```python
from build123d import *

# Parameters (mm, degrees)
CROQUIS1_W              = 70
CROQUIS1_H              = 117
SALIENTE_EXTRUIR1_DEPTH = 5
CROQUIS2_W              = 70
CROQUIS2_H              = 11.75
SALIENTE_EXTRUIR2_DEPTH = 40
CROQUIS5_R              = 1
CORTAR_EXTRUIR3_DEPTH   = 118
CROQUIS3_W              = 43.35
CROQUIS3_H              = 81.55
CORTAR_EXTRUIR1_DEPTH   = 10
SALIENTE_EXTRUIR4_DEPTH = 40
CROQUIS7_R              = 1.25
CROQUIS7_W              = 60
CROQUIS7_H              = 11.191024472
CORTAR_EXTRUIR5_DEPTH   = 71
CROQUIS9_W              = 50
CROQUIS9_H              = 20
CORTAR_EXTRUIR6_DEPTH   = 118
CROQUIS11_W             = 5
CROQUIS11_H             = 45
CROQUIS11_H_2           = 15
CROQUIS11_H_3           = 10
SALIENTE_EXTRUIR5_DEPTH = 20
CROQUIS12_W             = 42.5
CROQUIS12_H             = 15
CORTAR_EXTRUIR7_DEPTH   = 20
CROQUIS13_W             = 5
CROQUIS13_H             = 31.75
SALIENTE_EXTRUIR6_DEPTH = 5
CROQUIS14_W             = 55
CROQUIS14_H             = 31.75
SALIENTE_EXTRUIR7_DEPTH = 5


with BuildPart() as part:
    # Croquis1 → Saliente-Extruir1 (new body)
    with BuildSketch(Plane(origin=(0, 0, 0), x_dir=(1, 0, 0), z_dir=(0, 1, 0))):
        Rectangle(CROQUIS1_W, CROQUIS1_H)
    extrude(amount=SALIENTE_EXTRUIR1_DEPTH)

    # Croquis2 → Saliente-Extruir2 (add)
    with BuildSketch(Plane(origin=(0, 5, 0), x_dir=(1, 0, 0), z_dir=(0, 1, 0))):
        with Locations((0, 52.625)):
            Rectangle(CROQUIS2_W, CROQUIS2_H)
        with Locations((0, -52.625)):
            Rectangle(CROQUIS2_W, CROQUIS2_H)
    extrude(amount=SALIENTE_EXTRUIR2_DEPTH)

    # Croquis5 → Cortar-Extruir3 (cut, through all)
    with BuildSketch(Plane(origin=(0, 0, -58.5), x_dir=(-1, 0, 0), z_dir=(0, 0, -1))):
        with Locations((5, 35)):
            Circle(CROQUIS5_R)
    extrude(amount=-CORTAR_EXTRUIR3_DEPTH, mode=Mode.SUBTRACT)

    # Croquis3 → Cortar-Extruir1 (cut)
    with BuildSketch(Plane(origin=(0, 5, 0), x_dir=(1, 0, 0), z_dir=(0, 1, 0))):
        with Locations((0, 10.775)):
            Rectangle(CROQUIS3_W, CROQUIS3_H)
    extrude(amount=-CORTAR_EXTRUIR1_DEPTH, mode=Mode.SUBTRACT)

    # Croquis8 → Saliente-Extruir4 (add)
    with BuildSketch(Plane(origin=(0, 5, 0), x_dir=(1, 0, 0), z_dir=(0, 1, 0))):
        Polygon((35, -46.75), (35, 46.75), (21.675, 46.75), (21.675, -30), (-21.675, -30), (-21.675, 46.75), (-35, 46.75), (-35, -46.75), align=None)
    extrude(amount=SALIENTE_EXTRUIR4_DEPTH)

    # Croquis7 → Cortar-Extruir5 (cut, through all)
    with BuildSketch(Plane.ZY.offset(35)):
        with Locations((-9.99, 32.49)):
            Circle(CROQUIS7_R)
        with Locations((9.99, 32.49)):
            Circle(CROQUIS7_R)
        with Locations((9.99, 12.51)):
            Circle(CROQUIS7_R)
        with Locations((-9.99, 12.51)):
            Circle(CROQUIS7_R)
        with Locations((-10.75, 23.745325958)):
            Rectangle(CROQUIS7_W, CROQUIS7_H)
    extrude(amount=-CORTAR_EXTRUIR5_DEPTH, mode=Mode.SUBTRACT)

    # Croquis9 → Cortar-Extruir6 (cut, through all)
    with BuildSketch(Plane.XY.offset(58.5)):
        with Locations((0, 20)):
            Rectangle(CROQUIS9_W, CROQUIS9_H)
    extrude(amount=-CORTAR_EXTRUIR6_DEPTH, mode=Mode.SUBTRACT)

    # Croquis11 → Saliente-Extruir5 (add)
    with BuildSketch(Plane(origin=(0, 0, -58.5), x_dir=(-1, 0, 0), z_dir=(0, 0, -1))):
        with Locations((30, 22.5)):
            Rectangle(CROQUIS11_W, CROQUIS11_H)
        with Locations((-20, 37.5)):
            Rectangle(CROQUIS11_W, CROQUIS11_H_2)
        with Locations((-20, 5)):
            Rectangle(CROQUIS11_W, CROQUIS11_H_3)
    extrude(amount=SALIENTE_EXTRUIR5_DEPTH)

    # Croquis12 → Cortar-Extruir7 (cut)
    with BuildSketch(Plane(origin=(0, 0, -58.5), x_dir=(-1, 0, 0), z_dir=(0, 0, -1))):
        with Locations((3.75, 37.5)):
            Rectangle(CROQUIS12_W, CROQUIS12_H)
    extrude(amount=-CORTAR_EXTRUIR7_DEPTH, mode=Mode.SUBTRACT)

    # Croquis13 → Saliente-Extruir6 (add)
    with BuildSketch(Plane(origin=(0, 45, 0), x_dir=(1, 0, 0), z_dir=(0, 1, 0))):
        Polygon((-32.5, 78.5), (-27.5, 78.5), (-27.5, 58.5), (-25, 58.5), (-25, 46.75), (-32.5, 46.75), align=None)
        with Locations((20, 62.625)):
            Rectangle(CROQUIS13_W, CROQUIS13_H)
    extrude(amount=SALIENTE_EXTRUIR6_DEPTH)

    # Croquis14 → Saliente-Extruir7 (add)
    with BuildSketch(Plane(origin=(0, 50, 0), x_dir=(1, 0, 0), z_dir=(0, 1, 0))):
        with Locations((-5, 62.625)):
            Rectangle(CROQUIS14_W, CROQUIS14_H)
    extrude(amount=SALIENTE_EXTRUIR7_DEPTH)


solid = part.part
```
Can you work these out from the model? Positions are in its coordinate system, mm. A direction names the side the tool comes from. Coordinates: 2 decimals unless noted, no trailing zeros. Loops run counter-clockwise (first coordinate to the right, second up) from the corner with the lowest first, then second, coordinate; pieces in that order, holes last.
1) Imagine slicing it at B-B on y = 6.5. List the corners of the cut face in (x, z) for me (3 decimals), plus the area to 3 significant figures.
2) Imagine slicing it at A-A on z = -60.5. List the corners of the cut face in (x, y) for me.
3) For pin 1 (1 mm diameter, centred on x = -10.5, z = 31.5, fed in from +Y); pin 2 (12.5 mm diameter, centred on y = 42.5, z = -68.5, fed in from +X); pin 3 (2 mm diameter, centred on y = 47.5, z = -38.5, fed in from -X); pin 4 (4 mm diameter, centred on x = 18, y = 47.5, fed in from +Z), each with a flat end and sliding along its axis, tell me the tip position at first contact or that it passes through.
4) I need wall thicknesses on probe 1 along X at (y, z) = (33, -23) (3 decimals); probe 2 along Y at (x, z) = (-24.5, 52.5); probe 3 along Z at (x, y) = (21.5, 43.5). Which ranges of each line are inside material? Lowest first, please.
5) Imagine slicing it at D-D on z = -37. List the corners of the cut face in (x, y) for me (3 decimals).
6) Which directions (+Z, -Z, +X, -X, +Y, -Y) give clear straight access to the entire face, cutting with the end or side of a thin tool? Please do faces 1 (the flat face through (30, 18.15, -11)), 2 (the flat face through (21.675, 37, -9)), 3 (the flat face through (22, 10, 6)), 4 (the flat face through (-25, 29.7, -0.8)).
7) Imagine slicing it at C-C on x = 11.5. List the corners of the cut face in (y, z) for me, plus the area to 3 significant figures.
8) Thinking about a two-plate mould opening in Z: for faces 5 (the flat face through (-5, 50, -63)), 6 (the flat face through (-30, 18.15, -11)), 7 (the cylindrical face through (-30.07, 12.89, -8.8)), which applies, pulls with the +Z half, pulls with the -Z half, needs draft (parallel to the pull), parting line crosses it, or undercut?
Completed:
1. outline: (-35, -58.5) - (-32.5, -58.5) - (-32.5, -78.5) - (-27.5, -78.5) - (-27.5, -58.5) - (17.5, -58.5) - (17.5, -78.5) - (22.5, -78.5) - (22.5, -58.5) - (35, -58.5) - (35, 58.5) - (-35, 58.5) - close; hole (-21.675, -46.75) - (21.675, -46.75) - (21.675, 30) - (-21.675, 30) - close
1. area: 5,060 mm2
2. outline: (-32.5, 0) - (-27.5, 0) - (-27.5, 50) - (17.5, 50) - (17.5, 30) - (22.5, 30) - (22.5, 55) - (-32.5, 55) - close; (17.5, 0) - (22.5, 0) - (22.5, 10) - (17.5, 10) - close
3. pin 1: stops at y = 45
3. pin 2: stops at x = 22.5
3. pin 3: passes through
3. pin 4: stops at z = -46.75
4. probe 1: x = -35 to -21.675, 21.675 to 35
4. probe 2: y = 0 to 10, 30 to 45
4. probe 3: z = -78.5 to -46.75, 30 to 58.5
5. outline: (-35, 0) - (-21.675, 0) - (-21.675, 10) - (-25, 10) - (-25, 18.15) - (-35, 18.15) - close; (-35, 29.341) - (-25, 29.341) - (-25, 30) - (-21.675, 30) - (-21.675, 45) - (-35, 45) - close; (21.675, 0) - (35, 0) - (35, 18.15) - (25, 18.15) - (25, 10) - (21.675, 10) - close; (21.675, 30) - (25, 30) - (25, 29.341) - (35, 29.341) - (35, 45) - (21.675, 45) - close
6. face 1: +X, -X
6. face 2: +Y, -Y
6. face 3: +Z, -Z
6. face 4: -Z
7. outline: (0, -58.5) - (10, -58.5) - (10, -46.75) - (5, -46.75) - (5, -51.55) - (0, -51.55) - close; (0, 30) - (10, 30) - (10, 58.5) - (0, 58.5) - close; (30, 30) - (45, 30) - (45, 58.5) - (30, 58.5) - close; (50, -78.5) - (55, -78.5) - (55, -46.75) - (50, -46.75) - close
7. area: 965 mm2
8. face 5: needs draft
8. face 6: undercut
8. face 7: undercut
